```python
from build123d import *

# Parameters (mm, degrees)
SKETCH6_R           = 6.123610741
BOSS_EXTRUDE1_DEPTH = 4
SKETCH1_R           = 1.5
SKETCH1_R_2         = 4.75
CUT_EXTRUDE1_DEPTH  = 34.832676052
SKETCH4_R           = 2.5
CUT_EXTRUDE2_DEPTH  = 34.832676052


with BuildPart() as part:
    # Sketch6 → Boss-Extrude1 (new body)
    with BuildSketch(Plane.XY):
        with BuildLine():
            ThreePointArc((-13.876389259, 15), (-20, 8.876389259), (-26.123610741, 15))
            Line((-26.123610741, 15), (-26.123610741, -15))
            ThreePointArc((-26.123610741, -15), (-20, -8.876389259), (-13.876389259, -15))
            ThreePointArc((-13.876389259, -15), (-14.744302684, -18.142650827), (-17.102020228, -20.394471406))
            ThreePointArc((-17.102020228, -20.394471406), (0, -16.091558121), (17.102020228, -20.394471406))
            ThreePointArc((17.102020228, -20.394471406), (16.857349173, -9.744302684), (26.123610741, -15))
            Line((26.123610741, -15), (26.123610741, 15))
            ThreePointArc((26.123610741, 15), (16.857349173, 9.744302684), (17.102020228, 20.394471406))
            ThreePointArc((17.102020228, 20.394471406), (0, 16.091558121), (-17.102020228, 20.394471406))
            ThreePointArc((-17.102020228, 20.394471406), (-14.744302684, 18.142650827), (-13.876389259, 15))
        make_face()
        with Locations((-20, -15)):
            Circle(SKETCH6_R)
        with Locations((-20, 15)):
            Circle(SKETCH6_R)
        with Locations((20, 15)):
            Circle(SKETCH6_R)
        with Locations((20, -15)):
            Circle(SKETCH6_R)
    extrude(amount=BOSS_EXTRUDE1_DEPTH)

    # Sketch1 → Cut-Extrude1 (cut, through all)
    with BuildSketch(Plane.XY):
        with Locations((-8.75, -8.75)):
            Circle(SKETCH1_R)
        with Locations((-8.75, 8.75)):
            Circle(SKETCH1_R)
        with Locations((8.75, 8.75)):
            Circle(SKETCH1_R)
        with Locations((8.75, -8.75)):
            Circle(SKETCH1_R)
        Circle(SKETCH1_R_2)
    extrude(amount=CUT_EXTRUDE1_DEPTH, mode=Mode.SUBTRACT)

    # Sketch4 → Cut-Extrude2 (cut, through all)
    with BuildSketch(Plane.XY):
        with Locations((-20, 15)):
            Circle(SKETCH4_R)
        with Locations((20, 15)):
            Circle(SKETCH4_R)
        with Locations((20, -15)):
            Circle(SKETCH4_R)
        with Locations((-20, -15)):
            Circle(SKETCH4_R)
    extrude(amount=CUT_EXTRUDE2_DEPTH, mode=Mode.SUBTRACT)


solid = part.part
```
CAD build for the part. Positions are in the model's coordinates, mm. Coordinates: 2 decimals unless noted, no trailing zeros. Write each loop counter-clockwise with the first axis right and the second up, starting at its lowest first coordinate (ties: lowest second). Pieces come first, ordered by that corner, then holes. Notation, with made-up numbers: (-29.75, 45.5) -> (28.25, 45.5) arc R10 ccw to (28.25, 51.5) -> close; hole circle Ø7 at (66.5, 23). An arc over 180 degrees is marked (long way). Return JSON: item names as keys, results as strings. Group by question number.
Q1. Cut at C-C, the plane z = 2.15. State how many separate pieces and enclosed holes the cut face has, then the cut area to 3 significant figures.
Q2. Cut at A-A, the plane x = -20. Give the cut face in (y, z).
Q3. Drill centre lines: line 1 (X direction, y = -15, z = 1.3); line 2 (X direction, y = -8.75, z = 2.8); line 3 (Y direction, x = -20, z = 1.6). Where is each one in solid material? Low to high.
Q4. Cut at B-B, the plane y = 0. Give the cut face in (x, z), then the cut area to 3 significant figures.
Q5. Flat gauge pin, fed straight in: pin 1 (4.5 mm diameter, centred on x = -20, y = 15, fed in from +Z). Where does the tip first touch, or does it go through?
Q6. Cut at D-D, the plane y = -8.75. Give the cut face in (x, z).
Q7. Pull direction Y, two halves, no side cores. Call faces 1 (the face through (0, 5, 0)), 2 (the face through (-0.249, -16.092, 1.972)), 3 (the face through (-22.5, 15.1, 2)): released by +Y, released by -Y, zero draft, split by the parting line, or undercut.
Returned:
{
 "1": {"separate pieces": "1", "enclosed holes": "9", "area": "1,750 mm2"},
 "2": {"outline": "(-21.12, 0) -> (-17.5, 0) -> (-17.5, 4) -> (-21.12, 4) -> close; (-12.5, 0) -> (12.5, 0) -> (12.5, 4) -> (-12.5, 4) -> close; (17.5, 0) -> (21.12, 0) -> (21.12, 4) -> (17.5, 4) -> close"},
 "3": {"line 1": "x = -26.12 to -22.5, -17.5 to 17.5, 22.5 to 26.12", "line 2": "x = -26.12 to -10.25, -7.25 to 7.25, 10.25 to 26.12", "line 3": "y = -21.12 to -17.5, -12.5 to 12.5, 17.5 to 21.12"},
 "4": {"outline": "(-26.12, 0) -> (-4.75, 0) -> (-4.75, 4) -> (-26.12, 4) -> close; (4.75, 0) -> (26.12, 0) -> (26.12, 4) -> (4.75, 4) -> close", "area": "171 mm2"},
 "5": {"pin 1": "passes through"},
 "6": {"outline": "(-26.12, 0) -> (-10.25, 0) -> (-10.25, 4) -> (-26.12, 4) -> close; (-7.25, 0) -> (7.25, 0) -> (7.25, 4) -> (-7.25, 4) -> close; (10.25, 0) -> (26.12, 0) -> (26.12, 4) -> (10.25, 4) -> close"},
 "7": {"face 1": "zero draft", "face 2": "released by -Y", "face 3": "undercut"}
}
